Geometry check sheet. Reference: the model listing, model coordinates, mm. A direction names the side the tool comes from. Coordinates: 2 decimals unless noted, no trailing zeros. Write each loop counter-clockwise with the first axis right and the second up, starting at its lowest first coordinate (ties: lowest second). Pieces come first, ordered by that corner, then holes. Notation, with made-up numbers: (7.5, -24.5) -> (56.5, -24.5) arc R8 ccw to (56.5, -11.5) -> close; hole circle Ø10 at (-17, -15). An arc over 180 degrees is marked (long way). One line per question, with ' | ' between items.
from build123d import *


with BuildPart() as part:
    # Sketch2 → Revolve1 (revolve)
    with BuildSketch(Plane(origin=(0, 0, 0), x_dir=(0, 0, -1), z_dir=(1, 0, 0)), mode=Mode.PRIVATE) as revolve1_sk:
        with BuildLine():
            Line((20.0025, 27.432), (17.388963494, 27.432))
            ThreePointArc((17.388963494, 27.432), (17.084582779, 27.32867667), (16.906000581, 27.061409523))
            Line((16.906000581, 27.061409523), (14.418444847, 17.777725139))
            ThreePointArc((14.418444847, 17.777725139), (14.291807056, 17.556374904), (14.072477617, 17.426268585))
            Line((14.072477617, 17.426268585), (-14.920169656, 9.16644804))
            ThreePointArc((-14.920169656, 9.16644804), (-15.30374952, 9.212347173), (-15.540128252, 9.517904594))
            Line((-15.540128252, 9.517904594), (-16.906000581, 14.615409523))
            ThreePointArc((-16.906000581, 14.615409523), (-17.084582779, 14.88267667), (-17.388963494, 14.986))
            Line((-17.388963494, 14.986), (-20.0025, 14.986))
            Line((-20.0025, 14.986), (-20.0025, 8.636))
            Line((-20.0025, 8.636), (-17.3863, 8.636))
            Line((-17.3863, 8.636), (-17.3863, 7.874))
            Line((-17.3863, 7.874), (-13.431030881, 7.874))
            Line((-13.431030881, 7.874), (17.3863, 16.653661283))
            Line((17.3863, 16.653661283), (17.3863, 20.6502))
            Line((17.3863, 20.6502), (20.0025, 20.6502))
            Line((20.0025, 20.6502), (20.0025, 27.432))
        make_face()
    revolve(revolve1_sk.sketch.rotate(Axis((0, 0, 20.0025), (0, 0, -1)), 90), axis=Axis((0, 0, 20.0025), (0, 0, -1)))


solid = part.part
1. Cross-section at C-C on z = 0. Record the boundary of the cut face in (x, y), and give its area (3 significant figures).
Worked answers:
outline: circle Ø26.83 at (0, 0); hole circle Ø23.4 at (0, 0) | area: 135 mm²
2. Go/stop test with flat-tipped pins: P1, Ø2, axis at y = 1.5, z = -8.5, coming from the +X side; P2, Ø8.5, axis at x = -1, y = -4, coming from the +Z side; P3, Ø4, axis at x = -18.5, y = -11.5, coming from the +Z side; P4, Ø10.5, axis at x = 0, y = 0, coming from the -Z side. Record where each tip stops, or that it passes through.
Worked answers:
P1: x = 16.07 | P2: z = 17.39 | P3: z = -14.96 | P4: through
3. Tool access check on faces 4 (the face through (-1.124, -8.563, 18.676)), 5 (the face through (3.633, 6.986, 15.381)), 6 (the face through (-1, -17, -17.386)), 7 (the face through (-3.94, -20.45, -20.002)), 8 (the face through (9.383, -2.955, 15.626)). Record the directions out of +Z, -Z, +X, -X, +Y, -Y that give a thin tool (end or side, any length) a straight path to the whole face; none if there is none.
Worked answers:
face 4: +Z | face 5: +Z, -Z | face 6: -Z | face 7: -Z, +X, -X, +Y, -Y | face 8: none
4. Mould release check, pull along Y, two halves, no side actions. Record for faces 1 (the face through (14.294, -4.501, 18.714)), 2 (the face through (6.5, 6.5, 20.002)), 3 (the face through (10.826, -3.409, 1.231)): released by +Y, released by -Y, zero draft, split by the parting line, or undercut.
Worked answers:
face 1: split by the parting line | face 2: zero draft | face 3: undercut
5. Cross-section at D-D on z = -11. Record the boundary of the cut face in (x, y).
Worked answers:
outline: circle Ø33.1 at (0, 0); hole circle Ø29.67 at (0, 0)
6. Material ranges on line 1 (Y direction, x = 0, z = 18.3); line 2 (Y direction, x = 0, z = -18.55); line 3 (X direction, y = -6.5, z = 8), recorded low to high. Write a range as from..to.
Worked answers:
line 1: -14.99..-8.64, 8.64..14.99 | line 2: -27.43..-20.65, 20.65..27.43 | line 3: -9.04..-6.82, 6.82..9.04
